Design review of the part built by this model. Coordinates are the model's own, in mm. Face numbers are marked on the shaded views. Round coordinates to 2 decimals unless told otherwise and drop trailing zeros. Loops run counter-clockwise (first coordinate to the right, second up) from the corner with the lowest first, then second, coordinate; pieces in that order, holes last. Notation, with made-up numbers: (1, 76.25) -> (59, 76.25) arc R6 ccw to (59, 86.25) -> close; hole circle Ø1 at (61, 84.5). An arc over 180 degrees is marked (long way). Use a Markdown table: item, result. Add a question column.
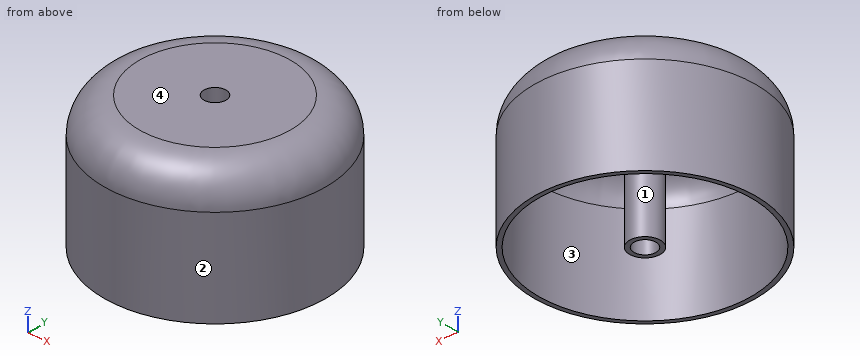
from build123d import *

# Parameters (mm, degrees)
F0_R     = 31.9398349348
F1_DEPTH = 38.1
F2_R     = 10.16
F4_D     = 6.35
F5_T     = -1.27


with BuildPart() as f1:
    # F0 (on Top) → F1 (new body)
    with BuildSketch(Plane.XY):
        Circle(F0_R)
    extrude(amount=F1_DEPTH)

    # F2
    f2_edges = [f1.edges().sort_by_distance(p)[0] for p in [
        (-31.939835, 0, 38.1),
    ]]
    fillet(f2_edges, radius=F2_R)

    # F4 (through all)
    with Locations(Plane.XY.offset(38.1)):
        with Locations((0, 0)):
            Hole(F4_D / 2)

    # F5
    f5_openings = [f1.faces().sort_by_distance(p)[0] for p in [
        (-31.03644, 0, 0),
    ]]
    offset(amount=F5_T, openings=f5_openings)


solid = f1.part
1. To check wall thickness, follow probe 1 along Z at (x, y) = (-19, 3); probe 2 along Y at (x, z) = (-13, 32.5); probe 3 along Y at (x, z) = (1.5, 22). State the ranges of each line that lie inside material, in increasing order. Write a range as from..to.
2. Insertion check: P1, Ø3, axis at y = 25, z = 7.5, coming from the +X side; P2, Ø3, axis at x = 4, y = -3, coming from the -Z side; P3, Ø2, axis at x = 8, z = 15, coming from the +Y side; P4, Ø10, axis at y = 13, z = 29.5, coming from the +X side. Each pin has a flat end and moves straight along its axis. Give the tip position at first contact, or say it passes through.
3. Consider section A-A on x = 0. State the section outline as (y, z) points (3 decimals), plus the area to 3 significant figures.
4. Consider section C-C on z = 2.5. State the section outline as (x, y) points (3 decimals), plus the area to 3 significant figures.
5. Mouldability with a two-part tool opening along Y and no side actions: class the marked faces 1, 2, 3 and 4 as +Y half, -Y half, draft (parallel to the pull), parting line (faces both ways), or undercut.
Verdict:
| question | item | result |
|---|---|---|
| 1 | probe 1 | z = 36.83..38.1 |
| 1 | probe 2 | y = -27.99..-26.38, 26.38..27.99 |
| 1 | probe 3 | y = -31.9..-30.63, -4.18..-2.8, 2.8..4.18, 30.63..31.9 |
| 2 | P1 | stops at x = 21.63 |
| 2 | P2 | stops at z = 0 |
| 2 | P3 | stops at y = 31.16 |
| 2 | P4 | stops at x = 30.88 |
| 3 | outline | (-31.94, 0) -> (-30.67, 0) -> (-30.67, 27.94) arc R8.89 cw to (-21.78, 36.83) -> (-4.445, 36.83) -> (-4.445, 0) -> (-3.175, 0) -> (-3.175, 38.1) -> (-21.78, 38.1) arc R10.16 ccw to (-31.94, 27.94) -> close; (3.175, 0) -> (4.445, 0) -> (4.445, 36.83) -> (21.78, 36.83) arc R8.89 cw to (30.67, 27.94) -> (30.67, 0) -> (31.94, 0) -> (31.94, 27.94) arc R10.16 ccw to (21.78, 38.1) -> (3.175, 38.1) -> close |
| 3 | area | 250 mm² |
| 4 | outline | circle Ø63.88 at (0, 0); circle Ø8.89 at (0, 0); hole circle Ø61.34 at (0, 0); hole circle Ø6.35 at (0, 0) |
| 4 | area | 280 mm² |
| 5 | face 1 | undercut |
| 5 | face 2 | parting line |
| 5 | face 3 | undercut |
| 5 | face 4 | draft |
